Check sheet for the modelled part. Datum: model origin and axes. Units: mm. A direction names the side the tool comes from. Round coordinates to 2 decimals unless told otherwise and drop trailing zeros. Order: outer loops, then holes, each group sorted by start corner. A loop starts at its lowest first (then second) coordinate and runs counter-clockwise, first axis right, second up. Notation, with made-up numbers: (-16.5, -26) -> (-5.5, -26) arc R25 cw to (-5.5, -4) -> close; hole circle Ø8 at (47, -32). An arc over 180 degrees is marked (long way). Answer in a Markdown table with one row per item.
```python
from build123d import *

# Parameters (mm, degrees)
SKETCH_W        = 31.8
SKETCH_H        = 15.8
PAD_DEPTH       = 9.6
SKETCH001_W     = 29.4
SKETCH001_H     = 13.4
POCKET_DEPTH    = 3.9
SKETCH002_R     = 2.4
PAD001_DEPTH    = 1.8
SKETCH003_R     = 2.4
PAD002_DEPTH    = 1.8
SKETCH004_R     = 2.4
PAD003_DEPTH    = 1.8
SKETCH005_R     = 2.4
PAD004_DEPTH    = 1.8
SKETCH006_R     = 3.25
PAD005_DEPTH    = 3.9
SKETCH007_R     = 2.4
POCKET001_DEPTH = 7.8
SKETCH008_R     = 3.25
PAD006_DEPTH    = 3.9
SKETCH009_R     = 2.4
POCKET002_DEPTH = 7.8


with BuildPart() as part:
    # Sketch → Pad (new body)
    with BuildSketch(Plane.XY):
        Rectangle(SKETCH_W, SKETCH_H)
    extrude(amount=PAD_DEPTH)

    # Sketch001 → Pocket (cut, symmetric)
    with BuildSketch(Plane.XY):
        Rectangle(SKETCH001_W, SKETCH001_H)
    extrude(amount=POCKET_DEPTH, both=True, mode=Mode.SUBTRACT)

    # Sketch002 (on Face5 of Pocket) → Pad001 (join)
    with BuildSketch(Plane.XY.offset(9.6)):
        with Locations((-12, 4)):
            Circle(SKETCH002_R)
    pad001 = extrude(amount=PAD001_DEPTH)

    # Sketch003 (on Face5 of Pad001) → Pad002 (join)
    with BuildSketch(Plane.XY.offset(9.6)):
        with Locations((-4, 4)):
            Circle(SKETCH003_R)
    pad002 = extrude(amount=PAD002_DEPTH)

    # Sketch004 (on Face5 of Pad002) → Pad003 (join)
    with BuildSketch(Plane.XY.offset(9.6)):
        with Locations((-12, -4)):
            Circle(SKETCH004_R)
    pad003 = extrude(amount=PAD003_DEPTH)

    # Sketch005 (on Face5 of Pad003) → Pad004 (join)
    with BuildSketch(Plane.XY.offset(9.6)):
        with Locations((-4, -4)):
            Circle(SKETCH005_R)
    pad004 = extrude(amount=PAD004_DEPTH)

    # Mirrored: Pad001, Pad002, Pad003, Pad004 across Sketch002 V_Axis
    add(pad001.mirror(Plane(origin=(0, 0, 9.6), x_dir=(0, 0, 1), z_dir=(1, 0, 0))))
    add(pad002.mirror(Plane(origin=(0, 0, 9.6), x_dir=(0, 0, 1), z_dir=(1, 0, 0))))
    add(pad003.mirror(Plane(origin=(0, 0, 9.6), x_dir=(0, 0, 1), z_dir=(1, 0, 0))))
    add(pad004.mirror(Plane(origin=(0, 0, 9.6), x_dir=(0, 0, 1), z_dir=(1, 0, 0))))

    # Sketch006 (on Face19 of Mirrored) → Pad005 (join, symmetric)
    with BuildSketch(Plane(origin=(0, 0, 3.9), x_dir=(1, 0, 0), z_dir=(0, 0, -1))):
        Circle(SKETCH006_R)
    extrude(amount=PAD005_DEPTH, both=True)

    # Sketch007 (on Face29 of Pad005) → Pocket001 (cut)
    with BuildSketch(Plane(origin=(0, 0, 0), x_dir=(1, 0, 0), z_dir=(0, 0, -1))):
        Circle(SKETCH007_R)
    extrude(amount=-POCKET001_DEPTH, mode=Mode.SUBTRACT)

    # Sketch008 (on Face19 of Pocket001) → Pad006 (join, symmetric)
    with BuildSketch(Plane(origin=(0, 0, 3.9), x_dir=(1, 0, 0), z_dir=(0, 0, -1))):
        with Locations((-8, 0)):
            Circle(SKETCH008_R)
    pad006 = extrude(amount=PAD006_DEPTH, both=True)

    # Sketch009 (on Face30 of Pad006) → Pocket002 (cut)
    with BuildSketch(Plane(origin=(0, 0, 0), x_dir=(1, 0, 0), z_dir=(0, 0, -1))):
        with Locations((-8, 0)):
            Circle(SKETCH009_R)
    pocket002 = extrude(amount=-POCKET002_DEPTH, mode=Mode.SUBTRACT)

    # Mirrored001: Pad006 across Sketch008 V_Axis
    add(pad006.mirror(Plane(origin=(0, 0, 3.9), x_dir=(0, 0, -1), z_dir=(1, 0, 0))))

    # Mirrored002: Pocket002 across Sketch009 V_Axis
    add(pocket002.mirror(Plane(origin=(0, 0, 0), x_dir=(0, 0, -1), z_dir=(1, 0, 0))), mode=Mode.SUBTRACT)


solid = part.part
```
(1) Depth check by flat-ended pin: pin 1 Ø4 at (x, y) = (-8, 0) entering from +Z; pin 2 Ø1.4 at (x, y) = (8, 0.5) entering from -Z. Enter the tip coordinate at first touch or a pass-through.
Solutions:
| item | result |
|---|---|
| pin 1 | z = 9.6 |
| pin 2 | z = 7.8 |
(2) Draft check along X on faces 4 (the flat face through (12, 4, 11.4)), 5 (the cylindrical face through (1.29, -2.024, 3.845)), 6 (the flat face through (-15.9, 0, 5)). Enter one of: pulls with the +X half, pulls with the -X half, needs draft (parallel to the pull), parting line crosses it, or undercut.
Solutions:
| item | result |
|---|---|
| face 4 | needs draft |
| face 5 | undercut |
| face 6 | pulls with the -X half |
(3) Section check C-C on z = 4.5. Record the boundary of the cut face in (x, y).
Solutions:
| item | result |
|---|---|
| outline | (-15.9, -7.9) -> (15.9, -7.9) -> (15.9, 7.9) -> (-15.9, 7.9) -> close; hole circle Ø4.8 at (-8, 0); hole circle Ø4.8 at (0, 0); hole circle Ø4.8 at (8, 0) |
(4) Tool access check on faces 1 (the cylindrical face through (-14.398, 4.106, 10.487)), 2 (the flat face through (-1, -7, 0)), 3 (the flat face through (-14.7, 0, 2)). Record the directions out of +Z, -Z, +X, -X, +Y, -Y that give a thin tool (end or side, any length) a straight path to the whole face; none if there is none.
Solutions:
| item | result |
|---|---|
| face 1 | +Z |
| face 2 | -Z, +X, -X, +Y, -Y |
| face 3 | -Z |
(5) Section check B-B on x = -4. Record the boundary of the cut face in (y, z).
Solutions:
| item | result |
|---|---|
| outline | (-7.9, 0) -> (-6.7, 0) -> (-6.7, 3.9) -> (6.7, 3.9) -> (6.7, 0) -> (7.9, 0) -> (7.9, 9.6) -> (6.4, 9.6) -> (6.4, 11.4) -> (1.6, 11.4) -> (1.6, 9.6) -> (-1.6, 9.6) -> (-1.6, 11.4) -> (-6.4, 11.4) -> (-6.4, 9.6) -> (-7.9, 9.6) -> close |
(6) Section check D-D on y = 4. Record the boundary of the cut face in (x, z), plus the area to 3 significant figures.
Solutions:
| item | result |
|---|---|
| outline | (-15.9, 0) -> (-14.7, 0) -> (-14.7, 3.9) -> (14.7, 3.9) -> (14.7, 0) -> (15.9, 0) -> (15.9, 9.6) -> (14.4, 9.6) -> (14.4, 11.4) -> (9.6, 11.4) -> (9.6, 9.6) -> (6.4, 9.6) -> (6.4, 11.4) -> (1.6, 11.4) -> (1.6, 9.6) -> (-1.6, 9.6) -> (-1.6, 11.4) -> (-6.4, 11.4) -> (-6.4, 9.6) -> (-9.6, 9.6) -> (-9.6, 11.4) -> (-14.4, 11.4) -> (-14.4, 9.6) -> (-15.9, 9.6) -> close |
| area | 225 mm^2 |
(7) Section check A-A on z = 10.5. Record the boundary of the cut face in (x, y), plus the area to 3 significant figures.
Solutions:
| item | result |
|---|---|
| outline | circle Ø4.8 at (-12, -4); circle Ø4.8 at (-12, 4); circle Ø4.8 at (-4, -4); circle Ø4.8 at (-4, 4); circle Ø4.8 at (4, -4); circle Ø4.8 at (4, 4); circle Ø4.8 at (12, -4); circle Ø4.8 at (12, 4) |
| area | 145 mm^2 |
(8) Scan lines: probe 1 along X at (y, z) = (0, 4); probe 2 along Y at (x, z) = (11.5, 3.5); probe 3 along Y at (x, z) = (8, 4). Record each from-to range of solid material in increasing order. Write a range as from..to.
Solutions:
| item | result |
|---|---|
| probe 1 | -15.9..-10.4, -5.6..-2.4, 2.4..5.6, 10.4..15.9 |
| probe 2 | -7.9..-6.7, 6.7..7.9 |
| probe 3 | -7.9..-2.4, 2.4..7.9 |
